Check sheet for the modelled part. Datum: model origin and axes. Units: mm. A direction names the side the tool comes from. Give positions to 0.01 mm unless a question says otherwise; leave off trailing zeros. Order: outer loops, then holes, each group sorted by start corner. A loop starts at its lowest first (then second) coordinate and runs counter-clockwise, first axis right, second up.
Item 1: Material ranges on line 1 along X through (y, z) = (75, 3.25); line 2 along Y through (x, z) = (42.5, 4.25); line 3 along Y through (x, z) = (12, 2.5), recorded low to high.
Item 2: Gauge pin test, flat ends, axial feed: P1, Ø3, axis at x = 13, z = 4.5, coming from the +Y side; P2, Ø3, axis at y = 4, z = 2.5, coming from the -X side; P3, Ø3, axis at y = 86, z = 4.5, coming from the +X side. Record the tip position at first contact, or that the pin passes through.
Item 3: Release check for a two-part mould opening along X. For faces 1 (the flat face through (76, 88.9, 3)), 2 (the flat face through (247.65, 44, 3)), 3 (the flat face through (184.15, 3, 3)) record: released by +X, released by -X, zero draft, split by the parting line, or undercut.
Item 4: Access from +Z, -Z, +X, -X, +Y, -Y to the whole of each face (thin tool, end or side, straight path). Record for faces 4 (the flat face through (82.55, 86, 3)), 5 (the flat face through (244, 82.55, 3)), 6 (the flat face through (254, 9, 3)), 7 (the flat face through (3, 50.8, 3)), 8 (the flat face through (146.05, 3, 3)).
Item 5: Sectioned sample at A-A on x = 162.5. Record the boundary of the cut face in (y, z).
from build123d import *

# Parameters (mm, degrees)
SKETCH2_W           = 88.9
SKETCH2_H           = 6.35
BOSS_EXTRUDE1_DEPTH = 254
SKETCH3_W           = 6.35
SKETCH3_H           = 12.7
SKETCH3_W_2         = 12.7
SKETCH3_H_2         = 6.35
SKETCH3_W_3         = 19.05
SKETCH3_H_3         = 5.615455356
CUT_EXTRUDE1_DEPTH  = 254


with BuildPart() as part:
    # Sketch2 → Boss-Extrude1 (new body)
    with BuildSketch(Plane.YZ):
        with Locations((44.45, 3.175)):
            Rectangle(SKETCH2_W, SKETCH2_H)
    extrude(amount=BOSS_EXTRUDE1_DEPTH)

    # Sketch3 → Cut-Extrude1 (cut)
    with BuildSketch(Plane.XY.offset(6.35)):
        with Locations((3.175, 19.05)):
            Rectangle(SKETCH3_W, SKETCH3_H)
        with Locations((250.825, 19.05)):
            Rectangle(SKETCH3_W, SKETCH3_H)
        with Locations((3.175, 44.45)):
            Rectangle(SKETCH3_W, SKETCH3_H)
        with Locations((3.175, 69.85)):
            Rectangle(SKETCH3_W, SKETCH3_H)
        with Locations((250.825, 44.45)):
            Rectangle(SKETCH3_W, SKETCH3_H)
        with Locations((250.825, 69.85)):
            Rectangle(SKETCH3_W, SKETCH3_H)
        with Locations((88.9, 3.175)):
            Rectangle(SKETCH3_W_2, SKETCH3_H_2)
        with Locations((63.5, 3.175)):
            Rectangle(SKETCH3_W_2, SKETCH3_H_2)
        with Locations((114.3, 3.175)):
            Rectangle(SKETCH3_W_2, SKETCH3_H_2)
        with Locations((139.7, 3.175)):
            Rectangle(SKETCH3_W_2, SKETCH3_H_2)
        with Locations((165.1, 3.175)):
            Rectangle(SKETCH3_W_2, SKETCH3_H_2)
        with Locations((190.5, 3.175)):
            Rectangle(SKETCH3_W_2, SKETCH3_H_2)
        with Locations((215.9, 3.175)):
            Rectangle(SKETCH3_W_2, SKETCH3_H_2)
        with Locations((244.475, 3.175)):
            Rectangle(SKETCH3_W_3, SKETCH3_H_2)
        with Locations((88.9, 85.725)):
            Rectangle(SKETCH3_W_2, SKETCH3_H_2)
        with Locations((63.5, 85.725)):
            Rectangle(SKETCH3_W_2, SKETCH3_H_2)
        with Locations((114.3, 85.725)):
            Rectangle(SKETCH3_W_2, SKETCH3_H_2)
        with Locations((139.7, 85.725)):
            Rectangle(SKETCH3_W_2, SKETCH3_H_2)
        with Locations((165.1, 85.725)):
            Rectangle(SKETCH3_W_2, SKETCH3_H_2)
        with Locations((190.5, 85.725)):
            Rectangle(SKETCH3_W_2, SKETCH3_H_2)
        with Locations((215.9, 85.725)):
            Rectangle(SKETCH3_W_2, SKETCH3_H_2)
        with Locations((244.475, 85.725)):
            Rectangle(SKETCH3_W_3, SKETCH3_H_2)
        with Locations((38.1, 85.725)):
            Rectangle(SKETCH3_W_2, SKETCH3_H_2)
        with Locations((9.525, 85.725)):
            Rectangle(SKETCH3_W_3, SKETCH3_H_2)
        with Locations((9.525, 2.807727678)):
            Rectangle(SKETCH3_W_3, SKETCH3_H_3)
        with Locations((38.1, 3.175)):
            Rectangle(SKETCH3_W_2, SKETCH3_H_2)
    extrude(amount=-CUT_EXTRUDE1_DEPTH, mode=Mode.SUBTRACT)


solid = part.part
Report:
1. line 1: x = 6.35 to 247.65
1. line 2: y = 6.35 to 82.55
1. line 3: y = 5.62 to 82.55
2. P1: stops at y = 82.55
2. P2: stops at x = 19.05
2. P3: stops at x = 234.95
3. face 1: zero draft
3. face 2: released by +X
3. face 3: undercut
4. face 4: +Z, -Z, +Y
4. face 5: +Z, -Z, +X, +Y
4. face 6: +Z, -Z, +X, +Y, -Y
4. face 7: +Z, -Z, -X
4. face 8: +Z, -Z, -Y
5. outline: (6.35, 0) - (82.55, 0) - (82.55, 6.35) - (6.35, 6.35) - close
